Verification items for the finished model (mm, model axes). Round coordinates to 2 decimals unless told otherwise and drop trailing zeros. One line per item, written item: value. Start each with the question number.
Autodesk Inventor part; units mm, degrees
ref_plane "YZ Plane" through (0, 0, 0) normal (1, 0, 0) x (0, 1, 0)
ref_plane "XZ Plane" through (0, 0, 0) normal (0, 1, 0) x (-1, 0, 0)
ref_plane "XY Plane" through (0, 0, 0) normal (0, 0, 1) x (1, 0, 0)
sketch "Sketch1" plane through (0, 0, 0) normal (0, 1, 0) x (-1, 0, 0)
  line L0 (0, 0) -> (200, 0)
  line L1 (200, 0) -> (200, -200)
  line L2 (200, -200) -> (0, -200)
  line L3 (0, -200) -> (0, 0)
  dimension "d0" = 200
  dimension "d1" = 200
extrude "Extrusion1" add sketch "Sketch1" along normal blind 2
fillet "Fillet1" radius 20 4 edges at (-200, 1, 0) (0, 1, 0) (0, 1, -200) (-200, 1, -200)
sketch "Sketch4" plane through (0, 2, 0) normal (0, 1, 0) x (1, 0, 0)
  arc A0 (-20, 0) -> (0, 20) centre (-20, 20) ccw
  arc A1 (-200, 20) -> (-180, 0) centre (-180, 20) ccw
  arc A2 (0, 180) -> (-20, 200) centre (-20, 180) ccw
  arc A3 (-180, 200) -> (-200, 180) centre (-180, 180) ccw
  circle A4 centre (-20, 180) radius 2.5
  circle A5 centre (-180, 180) radius 2.5
  circle A6 centre (-180, 20) radius 2.5
  circle A7 centre (-20, 20) radius 2.5
  line L0 (-180, 0) -> (-20, 0)
  line L1 (0, 20) -> (0, 180)
  point P0 (0, 0)
  dimension "d19" = 5
  dimension "d20" = 5
  dimension "d21" = 5
  dimension "d22" = 5
extrude "Extrusion4" cut sketch "Sketch4" against normal blind 2
properties part number "Basequadrada" material "PPS Plastic"
1) Mould release check, pull along X, two halves, no side actions. Record for faces 1 (the cylindrical face through (-178.66, 1.01, -182.11)), 2 (the cylindrical face through (-20.33, 1.01, -182.48)), 3 (the cylindrical face through (-194.297, 1.014, -6.014)), 4 (the flat face through (-99, 2, -99)): pulls with the +X half, pulls with the -X half, needs draft (parallel to the pull), parting line crosses it, or undercut.
2) Thickness scan on line 1 (Z direction, x = -20, y = 1.3); line 2 (Z direction, x = -16, y = 0.7). Record the ranges inside material, lowest first.
3) Gauge pin test, flat end, axial feed: pin 1 Ø4.5 at (x, z) = (-20, -180) entering from +Y. Record the tip position at first contact, or that the pin passes through.
Results below:
1. face 1: undercut
1. face 2: undercut
1. face 3: pulls with the -X half
1. face 4: needs draft
2. line 1: z = -200 to -182.5, -177.5 to -22.5, -17.5 to 0
2. line 2: z = -199.6 to -0.4
3. pin 1: passes through
